Could you check a few things on this model? Use its own coordinates, in mm. A direction names the side the tool comes from. Coordinates: 2 decimals unless noted, no trailing zeros. Loops run counter-clockwise (first coordinate to the right, second up) from the corner with the lowest first, then second, coordinate; pieces in that order, holes last. Notation, with made-up numbers: (11, -23) -> (60, -23) arc R18 cw to (60, -3) -> close; hole circle Ø8 at (87.25, 78). An arc over 180 degrees is marked (long way). One line per question, with ' | ' between items. Start each with the question number.
(1) If I drill on line 1 along Y through (x, z) = (-8.5, 0); line 2 along X through (y, z) = (32, 0); line 3 along Y through (x, z) = (2, 0), over which ranges is the centre line in solid material (lowest first)?
(2) Which directions (+Z, -Z, +X, -X, +Y, -Y) give clear straight access to the entire face, cutting with the end or side of a thin tool? Please do faces 4 (the face through (-3.417, 29.948, -0.759)), 5 (the face through (0.3, -17.5, -20.8)), 6 (the face through (-24, -15, 21)).
(3) I'm going to push flat-ended pins straight in: pin 1 Ø10 at (x, z) = (17, -4) entering from -Y; pin 2 Ø2 at (x, y) = (-1, -12) entering from -Z; pin 3 Ø1 at (x, z) = (-2.5, 9.5) entering from +Y. Where does each tip first touch, or does it pass through?
(4) Suppose I cut it at C-C (x = -7.5). Please give me the cut outline in (y, z).
(5) Suppose I cut it at A-A (y = 0). Please give me the cut outline in (x, z).
(6) If we mould it in two halves opening along Y, with no side actions, what happens to faces 1 (the face through (24, -15, 21)), 2 (the face through (0, -21, 28)), 3 (the face through (-0.336, 21.036, 13.509))? For each: pulls with the +Y half, pulls with the -Y half, needs draft (parallel to the pull), parting line crosses it, or undercut.
(7) Suppose I cut it at B-B (z = 0). Please give me the cut outline in (x, y).
(8) Suppose I cut it at D-D (z = 17). Please give me the cut outline in (x, y).
```python
from build123d import *

# Parameters (mm, degrees)
SKETCH1_R           = 35
SKETCH1_R_2         = 25
BOSS_EXTRUDE1_DEPTH = 24
CUT_EXTRUDE2_DEPTH  = 69.949256704
SKETCH6_R           = 3.5
CUT_EXTRUDE3_DEPTH  = 24


with BuildPart() as part:
    # Sketch1 → Boss-Extrude1 (new, symmetric)
    with BuildSketch(Plane(origin=(0, 0, 0), x_dir=(0, 0, -1), z_dir=(1, 0, 0))):
        Circle(SKETCH1_R)
        Circle(SKETCH1_R_2, mode=Mode.SUBTRACT)
    extrude(amount=BOSS_EXTRUDE1_DEPTH, both=True)

    # Sketch5 → Cut-Extrude2 (cut, through all)
    with BuildSketch(Plane(origin=(24, 0, 0), x_dir=(0, 0, -1), z_dir=(1, 0, 0))):
        Polygon((22.080992746, -19.330798208), (10.612864126, -27.360868317), (2.618348192, -15.943516321), (14.086476812, -7.913446212), align=None)
    extrude(amount=-CUT_EXTRUDE2_DEPTH, mode=Mode.SUBTRACT)

    # Sketch6 → Cut-Extrude3 (cut)
    with BuildSketch(Plane(origin=(0, 35, 0), x_dir=(-1, 0, 0), z_dir=(0, 1, 0))):
        with Locations(Location((0, 0, 0), (0, 0, 90))):
            Circle(SKETCH6_R)
    extrude(amount=-CUT_EXTRUDE3_DEPTH, mode=Mode.SUBTRACT)


solid = part.part
```
Checks:
1) line 1: y = -35 to -25, 25 to 35 | line 2: x = -24 to -3.5, 3.5 to 24 | line 3: y = -35 to -25
2) face 4: +Y | face 5: +X, -X | face 6: +Z, -Z, -X, +Y, -Y
3) pin 1: stops at y = -35 | pin 2: stops at z = -33.23 | pin 3: stops at y = 33.82
4) outline: circle Ø70 at (0, 0); hole (-27.36, -10.61) -> (-19.33, -22.08) -> (-15.64, -19.5) arc R25 ccw (long way) to (-23.67, -8.03) -> close
5) outline: (-24, -35) -> (24, -35) -> (24, -25) -> (-24, -25) -> close; (-24, 25) -> (24, 25) -> (24, 35) -> (-24, 35) -> close
6) face 1: needs draft | face 2: parting line crosses it | face 3: undercut
7) outline: (-24, -35) -> (24, -35) -> (24, -25) -> (-24, -25) -> close; (-24, 25) -> (-3.5, 25) -> (-3.5, 35) -> (-24, 35) -> close; (3.5, 25) -> (24, 25) -> (24, 35) -> (3.5, 35) -> close
8) outline: (-24, -30.59) -> (24, -30.59) -> (24, -18.33) -> (-24, -18.33) -> close; (-24, 18.33) -> (24, 18.33) -> (24, 30.59) -> (-24, 30.59) -> close
